Print and shaded views of the part. All mm, measured from the part's lowest x, y and z. A direction names the side the tool comes from. Coordinates: 2 decimals unless noted, no trailing zeros. Loops run counter-clockwise (first coordinate to the right, second up) from the corner with the lowest first, then second, coordinate; pieces in that order, holes last. Notation, with made-up numbers: M 69,-20 L 112,-20 A19 ccw 112,-12 Z; hole C 57.5,60.5 d1. An arc over 180 degrees is marked long. Use a Markdown table: item, result. Add a question column.
1) Band-saw the part on A-A (z = 94.5). List the corners of the cut face in (x, y) (1 decimal).
2) Pin check, flat tips, straight feed: pin 1 Ø2 at (x, z) = (95.5, 39.5) entering from +Y; pin 2 Ø4 at (x, z) = (72.5, 118.5) entering from +Y; pin 3 Ø1.5 at (x, z) = (29.5, 110.5) entering from -Y. Stop position of each tip, or through.
3) Band-saw the part on B-B (z = 42). List the corners of the cut face in (x, y), plus the area to 3 significant figures.
4) Tool access for the marked faces 1 and 2: list every direction of +Z, -Z, +X, -X, +Y, -Y with a clear straight run to the whole face (end or side of a thin tool).
5) Wall check: probe 1 along X at (y, z) = (76, 125); probe 2 along X at (y, z) = (34.5, 47.5). Give the ranges that are in metal, low to high. Write a range as from..to.
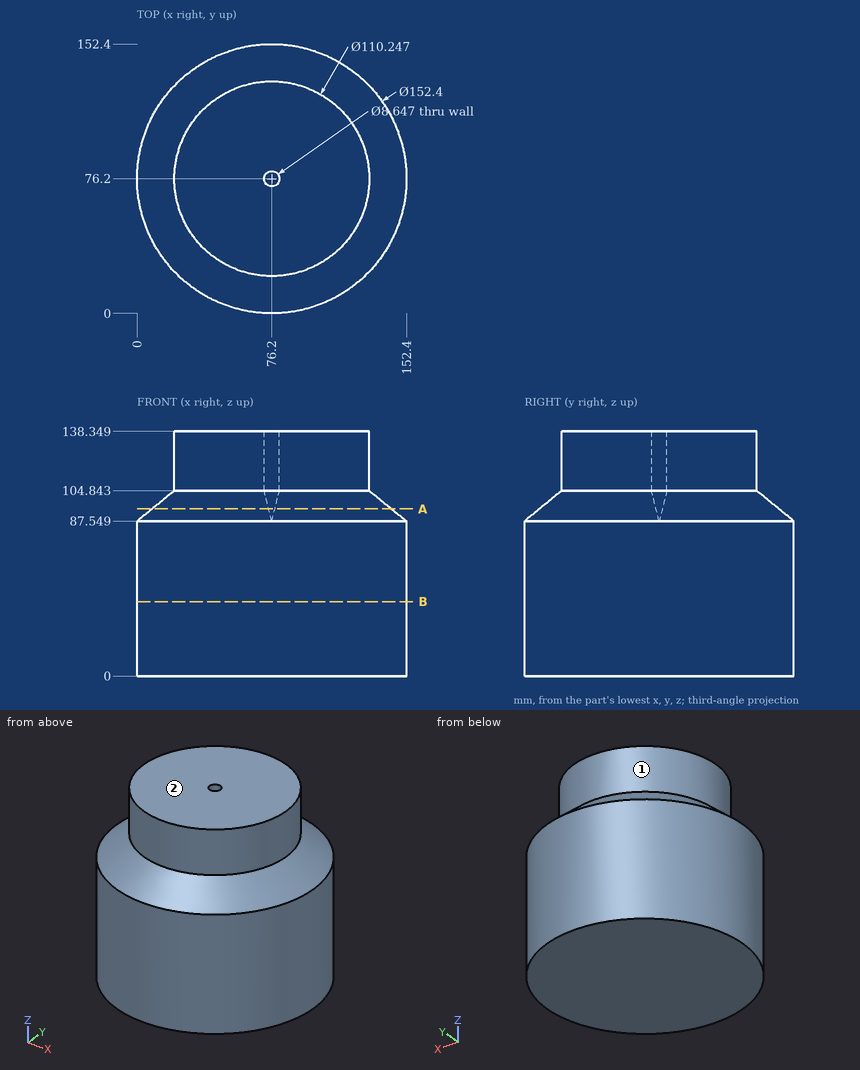
Entries:
| question | item | result |
|---|---|---|
| 1 | outline | C 76.2,76.2 d135.5; hole C 76.2,76.2 d3.5 |
| 2 | pin 1 | y = 150.17 |
| 2 | pin 2 | y = 131.3 |
| 2 | pin 3 | y = 45.75 |
| 3 | outline | C 76.2,76.2 d152.4 |
| 3 | area | 18,200 mm2 |
| 4 | face 1 | +Z |
| 4 | face 2 | +Z, +X, -X, +Y, -Y |
| 5 | probe 1 | 21.08..71.88, 80.52..131.32 |
| 5 | probe 2 | 12.42..139.98 |
